Read the model definition and answer for the solid it produces. Units are mm, in the model's axes. A direction names the side the tool comes from. Coordinates: 2 decimals unless noted, no trailing zeros. Order: outer loops, then holes, each group sorted by start corner. A loop starts at its lowest first (then second) coordinate and runs counter-clockwise, first axis right, second up. Notation, with made-up numbers: (43.5, 12.5) -> (92.5, 12.5) arc R20 cw to (92.5, 32.5) -> close; hole circle Ø3 at (-8.5, 58). An arc over 180 degrees is marked (long way). Use CSV: the item, a comma, the result in double quotes.
```python
from build123d import *

# Parameters (mm, degrees)
PAD_DEPTH              = 13.8
BOX002_W               = 3
BOX002_H               = 10
BOX002_DEPTH           = 3
CYLINDER001_R          = 1.5
CYLINDER001_DEPTH      = 9.7
CYLINDER001_ROLL_ANGLE = 90
CLONE_PLACEMENT_ANGLE  = 180


with BuildPart() as motorbody:
    # Sketch → Pad (new body)
    with BuildSketch(Plane.XZ):
        with BuildLine():
            Line((-45, 21.25), (-16.5, 21.25))
            Line((-16.5, 21.25), (-16.5, 23.65))
            Line((-16.5, 23.65), (-13.5, 23.65))
            Line((-13.5, 23.65), (-13.5, 22.5))
            Line((-13.5, 22.5), (0, 22.5))
            Line((0, 22.5), (0, 0))
            Line((-13.5, 0), (0, 0))
            Line((-13.5, -1.15), (-13.5, 0))
            Line((-13.5, -1.15), (-16.5, -1.15))
            Line((-16.5, -1.15), (-16.5, 1.25))
            Line((-16.5, 1.25), (-44.999948, 1.25))
            ThreePointArc((-45, 21.25), (-54.999971, 11.249974), (-44.999948, 1.25))
        make_face()
    extrude(amount=PAD_DEPTH)


with BuildPart() as cube001:
    # Box002 → Box002 (new body)
    with BuildSketch(Plane(origin=(-46.5, -23.7, 12.25), x_dir=(1, 0, 0), z_dir=(0, 0, 1))):
        with Locations((1.5, 5)):
            Rectangle(BOX002_W, BOX002_H)
    extrude(amount=BOX002_DEPTH)


with BuildPart() as clone_of_motor:
    # Cylinder001 → Cylinder001 (new body)
    with BuildSketch(Plane.XY):
        Circle(CYLINDER001_R)
    extrude(amount=CYLINDER001_DEPTH)


with BuildPart() as clone_of_motor_1:
    # Cylinder001 roll: moved
    add(clone_of_motor.part.rotate(Axis((0, 0, 0), (1, 0, 0)), CYLINDER001_ROLL_ANGLE))


with BuildPart() as clone_of_motor_2:
    # Cylinder001 placement: moved
    add(clone_of_motor_1.part.moved(Location((-45, -13.8, 11.25))))

    # Cut: cut Cube001
    add(cube001.part, mode=Mode.SUBTRACT)

    # Fusion001: union motorBody
    add(motorbody.part)


with BuildPart() as clone_of_motor_3:
    # Fusion001 placement: moved
    add(clone_of_motor_2.part.moved(Location((34.1, -23.1, -1.5))))


with BuildPart() as clone_of_motor_4:
    # Clone placement: moved
    add(clone_of_motor_3.part.moved(Location((0, 13, 19.5))).rotate(Axis((0, 13, 19.5), (1, 0, 0)), CLONE_PLACEMENT_ANGLE))


solid = clone_of_motor_4.part
```
Item 1: Straight lines are drawn through the part: line 1 along Y through (x, z) = (28, 3); line 2 along X through (y, z) = (44, -1); line 3 along Z through (x, y) = (28, 37.75). For each, find the intervals that lie inside material, in ascending order.
Return value:
line 1,"y = 36.1 to 49.9"
line 2,"x = 17.6 to 34.1"
line 3,"z = -1.5 to 21"
Item 2: A tool of negligible diameter and unlimited length cuts with its end or side. For faces 1 (the flat face through (17.6, 43, -1)), 2 (the flat face through (-11, 55, 8.75)), 3 (the flat face through (20.6, 42.9, 21.6)), 4 (the cylindrical face through (-10.95, 54.68, 11.25)), from which of +Z, -Z, +X, -X, +Y, -Y can it reach the whole face along a straight path? Write none if from no direction.
Return value:
face 1,"-Z, -X, +Y, -Y"
face 2,"-Z, +X, -X, +Y"
face 3,"+Z, +X, +Y, -Y"
face 4,"+Y"
Item 3: Each of these flat-tipped pins is pushed along its axis until it touches: P1, Ø0.7, axis at y = 44, z = 20.5, coming from the -X side; P2, Ø6, axis at y = 40.5, z = 8, coming from the -X side; P3, Ø1.1, axis at x = -11, y = 54, coming from the -Z side; P4, Ø7, axis at x = 6.5, y = 41, coming from the +Z side. Where does it stop, or does it pass through?
Return value:
P1,"stops at x = 17.6"
P2,"stops at x = -20.9"
P3,"stops at z = 8.75"
P4,"stops at z = 19.75"
Item 4: Find section C-C, the plane x = -2. Give the vertices of the cut face in (y, z).
Return value:
outline,"(36.1, -0.25) -> (49.9, -0.25) -> (49.9, 19.75) -> (36.1, 19.75) -> close"
Item 5: Find section D-D, the plane y = 56. Give the vertices of the cut face in (x, z).
Return value:
outline,"(-12.02, 8.75) -> (-9.78, 8.75) arc R1.5 ccw (long way) to start"
Item 6: Find section B-B, the plane y = 45.25. Give the vertices of the cut face in (x, z), then the cut area to 3 significant figures.
Return value:
outline,"(-10.9, -0.25) -> (17.6, -0.25) -> (17.6, -2.65) -> (20.6, -2.65) -> (20.6, -1.5) -> (34.1, -1.5) -> (34.1, 21) -> (20.6, 21) -> (20.6, 22.15) -> (17.6, 22.15) -> (17.6, 19.75) -> (-10.9, 19.75) arc R10 ccw to start"
area,"1,110 mm^2"
Item 7: Find section A-A, the plane z = 9.75. Give the vertices of the cut face in (x, y).
Return value:
outline,"(-20.9, 36.1) -> (34.1, 36.1) -> (34.1, 49.9) -> (-9.4, 49.9) -> (-9.4, 59.6) -> (-12.4, 59.6) -> (-12.4, 49.9) -> (-20.9, 49.9) -> close"
